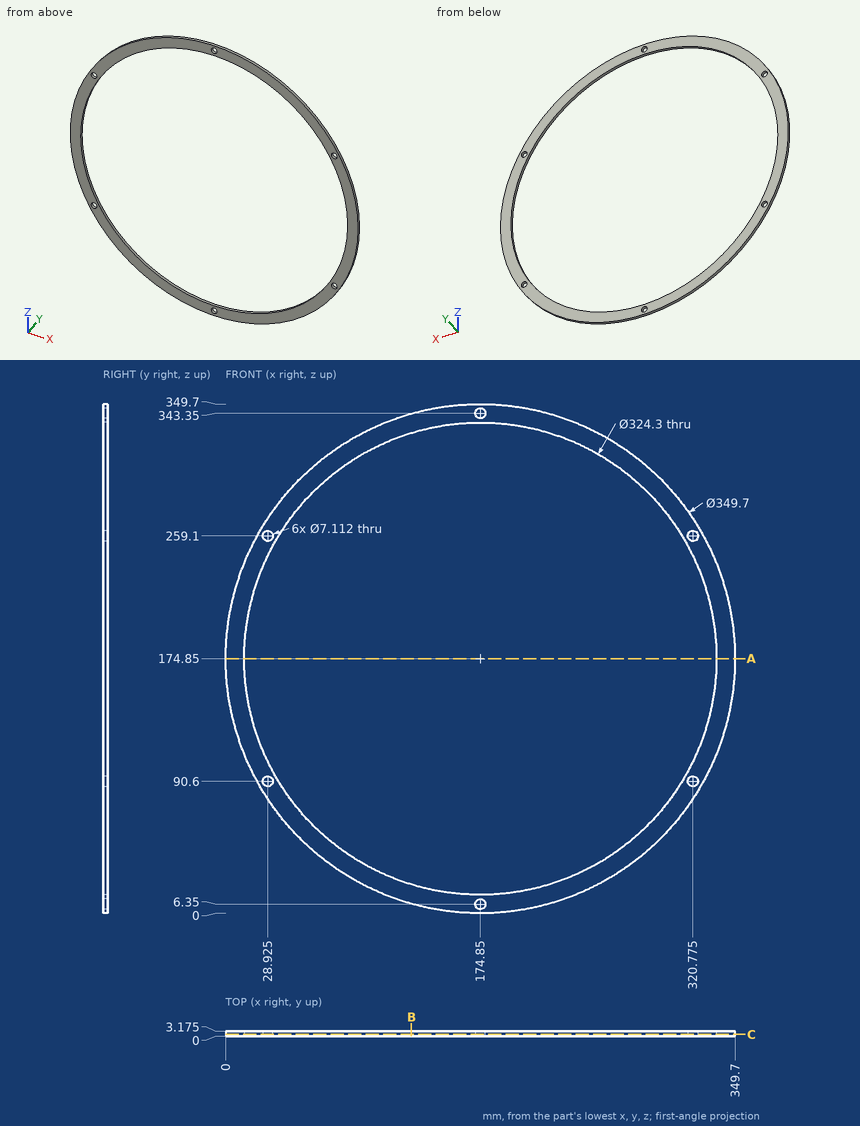
Check sheet for the drawn part. Datum: minimum x, y, z corner. Units: mm. Give positions to 0.01 mm unless a question says otherwise; leave off trailing zeros. Write each loop counter-clockwise with the first axis right and the second up, starting at its lowest first coordinate (ties: lowest second). Pieces come first, ordered by that corner, then holes. Notation, with made-up numbers: M 39.5,48.5 L 86.5,48.5 A13 cw 86.5,61.5 Z; hole C -9.5,56 d2. An arc over 180 degrees is marked long. One line per question, with ' | ' between items.
1) Gauge pin test, flat ends, axial feed: pin 1 Ø1 at (x, y) = (80.5, 1) entering from +Z; pin 2 Ø8 at (x, z) = (28.92, 259.1) entering from +Y (3 decimals). Record the tip position at first contact, or that the pin passes through.
Result:
pin 1: stops at z = 322.38 | pin 2: stops at y = 3.175
2) Section check A-A on z = 174.85. Enter the section's corners in (x, y) (1 decimal).
Result:
outline: M 0,0 L 12.7,0 L 12.7,3.2 L 0,3.2 Z; M 337,0 L 349.7,0 L 349.7,3.2 L 337,3.2 Z
3) Section check B-B on x = 127.5. Enter the section's corners in (y, z) (1 decimal).
Result:
outline: M 0,6.5 L 3.2,6.5 L 3.2,19.8 L 0,19.8 Z; M 0,329.9 L 3.2,329.9 L 3.2,343.2 L 0,343.2 Z
4) Section check C-C on y = 1.1. State how many separate pieces and enclosed holes the cut face has, plus the area to 3 significant figures.
Result:
separate pieces: 1 | enclosed holes: 7 | area: 13,200 mm2
5) Thickness scan on line 1 along X through (y, z) = (2.05, 174); line 2 along X through (y, z) = (0.9, 182.5); line 3 along Z through (x, y) = (218.5, 1.7) (1 decimal). Record the ranges inside material, lowest first. Write a range as [from, to].
Result:
line 1: x = [0, 12.7], [337, 349.7] | line 2: x = [0.17, 12.88], [336.82, 349.53] | line 3: z = [5.5, 18.7], [331, 344.2]
